Here's how the part is built. I have some questions about the finished solid (model axes, mm). A direction names the side the tool comes from. Coordinates: 2 decimals unless noted, no trailing zeros. Loops run counter-clockwise (first coordinate to the right, second up) from the corner with the lowest first, then second, coordinate; pieces in that order, holes last. Notation, with made-up numbers: (52.5, 52.5) -> (106.5, 52.5) arc R19 ccw to (106.5, 80.5) -> close; hole circle Ø3 at (16, 87). An arc over 180 degrees is marked (long way). Answer as a JSON object with one key per item and string values. Group by question number.
Q1. I want a section at C-C on y = 2.5. Write out the boundary of the cut face in (x, z).
Q2. I want a section at A-A on x = 0. Write out the boundary of the cut face in (y, z) (3 decimals).
Q3. I want a section at B-B on y = -1. Write out the boundary of the cut face in (x, z) (3 decimals).
Q4. I need wall thicknesses on line 1 (X direction, y = -1.55, z = 0) (3 decimals); line 2 (Z direction, x = 0, y = -1.45) (3 decimals); line 3 (Y direction, x = -4, z = -1). Which ranges of each line are inside material? Lowest first, please.
Q5. On a 3-axis mill with a long thin cutter (end or side, diameter ignored), from which of +Z, -Z, +X, -X, +Y, -Y can I reach the whole of each face in a straight line? I mean faces 1 (the cylindrical face through (0.1, 3, -3.5)), 2 (the flat face through (-1.8, 1, 5)), 3 (the cylindrical face through (0.32, -1.23, -7.85)). Say none if no direction works.
Q6. Thinking about a two-plate mould opening in Z: for faces 4 (the cylindrical face through (0, 0.9, -1.8)), 5 (the flat face through (-2.3, 4.3, -3.3)), 6 (the cylindrical face through (0.4, 0.76, -9.74)), 7 (the flat face through (1, 1.8, -2)), which applies, released by +Z, released by -Z, zero draft, split by the parting line, or undercut?
Q7. I'm going to push flat-ended pins straight in: pin 1 (8 mm diameter, centred on x = -5, z = -3.5, fed in from -Y); pin 2 (6.5 mm diameter, centred on x = -1, z = 0, fed in from -Y); pin 3 (3.5 mm diameter, centred on y = 0, z = 4.5, fed in from -X); pin 4 (1 mm diameter, centred on x = 7.5, y = 0.5, fed in from +Z). Where does each tip first touch, or does it pass through?
```python
from build123d import *

# Parameters (mm, degrees)
TAGLIO_ESTRUSIONE1_DEPTH = 16.374166644


with BuildPart() as part:
    # Schizzo1 → Rivoluzione1 (revolve)
    with BuildSketch(Plane.XY, mode=Mode.PRIVATE) as rivoluzione1_sk:
        with BuildLine():
            Line((0, 0), (-6.415, 0))
            Line((-6.415, 0), (-6.415, -2.5))
            Line((-6.415, -2.5), (-7.855, -2.5))
            Line((-7.855, -2.5), (-7.855, 0))
            Line((-7.855, 0), (-9.75, 0))
            Line((-9.75, 0), (-9.75, 1.5))
            ThreePointArc((-9.75, 1.5), (-6.993076896, 2.252094735), (-5, 4.3))
            Line((-5, 4.3), (-3.5, 4.3))
            Line((-3.5, 4.3), (-3.5, 1.8))
            Line((-3.5, 1.8), (0, 1.8))
            Line((0, 1.8), (0, 0))
        make_face()
    revolve(rivoluzione1_sk.sketch.rotate(Axis((0, -12.420504762, 0), (0, 1, 0)), 270), axis=Axis((0, -12.420504762, 0), (0, 1, 0)))

    # Schizzo2 → Taglio-Estrusione1 (cut, through all)
    with BuildSketch(Plane(origin=(0, 4.3, 0), x_dir=(1, 0, 0), z_dir=(0, 1, 0))):
        with BuildLine():
            Line((1.8, -9.582405752), (1.8, 0))
            ThreePointArc((1.8, 0), (0, 1.8), (-1.8, 0))
            Line((-1.8, 0), (-1.8, -9.582405752))
            ThreePointArc((-1.8, -9.582405752), (0, -9.75), (1.8, -9.582405752))
        make_face()
    extrude(amount=-TAGLIO_ESTRUSIONE1_DEPTH, mode=Mode.SUBTRACT)


solid = part.part
```
Result set:
{
 "1": {"outline": "(-1.8, 3) -> (-1.8, 6.36) arc R6.61 ccw (long way) to (1.8, 6.36) -> (1.8, 3) arc R3.5 cw (long way) to start"},
 "2": {"outline": "(-2.5, -7.855) -> (0, -7.855) -> (0, -9.75) -> (1.5, -9.75) arc R5.429 cw to (4.3, -5) -> (4.3, -3.5) -> (1.8, -3.5) -> (1.8, -1.8) -> (0, -1.8) -> (0, -6.415) -> (-2.5, -6.415) -> close"},
 "3": {"outline": "(-1.8, 6.157) -> (-1.8, 7.646) arc R7.855 ccw (long way) to (1.8, 7.646) -> (1.8, 6.157) arc R6.415 cw (long way) to start"},
 "4": {"line 1": "x = -7.855 to -6.415, 6.415 to 7.855", "line 2": "z = -7.855 to -6.415", "line 3": "y = 0 to 4.3"},
 "5": {"face 1": "+Y", "face 2": "+Z, +Y, -Y", "face 3": "-Y"},
 "6": {"face 4": "released by +Z", "face 5": "zero draft", "face 6": "split by the parting line", "face 7": "undercut"},
 "7": {"pin 1": "stops at y = -2.5", "pin 2": "stops at y = 0", "pin 3": "stops at x = -9.35", "pin 4": "stops at z = 6.79"}
}
